CAD build for the part. Positions are in the model's coordinates, mm. A direction names the side the tool comes from. Round coordinates to 2 decimals unless told otherwise and drop trailing zeros. Write each loop counter-clockwise with the first axis right and the second up, starting at its lowest first coordinate (ties: lowest second). Pieces come first, ordered by that corner, then holes. Notation, with made-up numbers: (-16.5, 29.5) - (-3.5, 29.5) arc R5 cw to (-3.5, 37.5) - close; hole circle Ø10 at (11.5, -18). An arc over 180 degrees is marked (long way). Answer in a Markdown table with one row per item.
```python
from build123d import *

# Parameters (mm, degrees)
F0_W     = 58.42
F0_H     = 58.42
F1_DEPTH = 68.390979
F2_W     = 34.69379
F2_H     = 28.147937
F4_R     = 13.288258
F5_DEPTH = 140.97


with BuildPart() as f1:
    # F0 (on Top) → F1 (new body)
    with BuildSketch(Plane.XY):
        with Locations((-12.080159, 8.183077)):
            Rectangle(F0_W, F0_H)
    extrude(amount=F1_DEPTH)

    # F2 (on face) → F3 (revolve)
    with BuildSketch(Plane.XZ.offset(21.026923)):
        with Locations((-14.097282, 32.681106)):
            Rectangle(F2_W, F2_H)
    revolve(axis=Axis((17.129841, -21.026923, 34.195489), (0, 0, 1)))

    # F4 (on face) → F5 (cut)
    with BuildSketch(Plane.XY.offset(68.390979)):
        with Locations((-23.98462, 13.432804)):
            Circle(F4_R)
    extrude(amount=-F5_DEPTH, mode=Mode.SUBTRACT)


solid = f1.part
```
Q1. Flat gauge pins, fed straight in: pin 1 (22 mm diameter, centred on x = 17.13, y = -21.03, fed in from -Z); pin 2 (17.5 mm diameter, centred on y = -1.5, z = 45, fed in from +X); pin 3 (8 mm diameter, centred on y = -2, z = 23, fed in from +X); pin 4 (1.5 mm diameter, centred on x = 32.5, y = 7.5, fed in from +Z). Where does each tip first touch, or does it go through?
Computed:
| item | result |
|---|---|
| pin 1 | stops at z = 0 |
| pin 2 | stops at x = 64.49 |
| pin 3 | stops at x = 63.32 |
| pin 4 | stops at z = 46.76 |
Q2. Saw through at A-A on x = -29. List the corners of the cut face in (y, z).
Computed:
| item | result |
|---|---|
| outline | (-36.24, 18.61) - (-21.03, 18.61) - (-21.03, 0) - (1.13, 0) - (1.13, 68.39) - (-21.03, 68.39) - (-21.03, 46.76) - (-36.24, 46.76) - close; (25.74, 0) - (37.39, 0) - (37.39, 68.39) - (25.74, 68.39) - close |
Q3. Pull direction X, two halves, no side cores. Call faces 1 (the cylindrical face through (-34.53, 5.35, 34.67)), 2 (the cylindrical face through (50.325, -56.488, 32.878)), 3 (the flat face through (-41.29, 8, 34)): released by +X, released by -X, zero draft, split by the parting line, or undercut.
Computed:
| item | result |
|---|---|
| face 1 | undercut |
| face 2 | split by the parting line |
| face 3 | released by -X |
Q4. Saw through at D-D on z = 30.5. List the corners of the cut face in (x, y), then the cut area to 3 significant figures.
Computed:
| item | result |
|---|---|
| outline | (-41.29, -21.03) - (-31.44, -21.03) arc R48.57 ccw (long way) to (17.13, 27.55) - (17.13, 37.39) - (-41.29, 37.39) - close; hole circle Ø26.58 at (-23.98, 13.43); hole (3.25, -21.03) arc R13.88 ccw (long way) to (17.13, -7.15) - (17.13, -21.03) - close |
| area | 7,960 mm2 |
Q5. Drill centre lines: line 1 (Z direction, x = 57, y = -34); line 2 (Y direction, x = -12, z = 63.5); line 3 (X direction, y = -31, z = 45). Where is each one in solid material? Low to high.
Computed:
| item | result |
|---|---|
| line 1 | z = 18.61 to 46.76 |
| line 2 | y = -21.03 to 7.69, 19.17 to 37.39 |
| line 3 | x = -30.41 to 7.48, 26.78 to 64.67 |
Q6. 3-axis set-ups, long thin cutter, end or side, ignore diameter. For faces 4 (the flat face through (29, -33, 46.755)), 5 (the flat face through (-12, 37.393, 34)), 6 (the flat face through (29, -33, 18.607)): which of +Z, -Z, +X, -X, +Y, -Y reach the whole face in a straight line?
Computed:
| item | result |
|---|---|
| face 4 | +Z, +X, -Y |
| face 5 | +Z, -Z, +X, -X, +Y |
| face 6 | -Z, +X, -Y |
Q7. Saw through at C-C on z = 4. List the corners of the cut face in (x, y), then the cut area to 3 significant figures.
Computed:
| item | result |
|---|---|
| outline | (-41.29, -21.03) - (17.13, -21.03) - (17.13, 37.39) - (-41.29, 37.39) - close; hole circle Ø26.58 at (-23.98, 13.43) |
| area | 2,860 mm2 |
Q8. Saw through at B-B on y = 12. List the corners of the cut face in (x, z), then the cut area to 3 significant figures.
Computed:
| item | result |
|---|---|
| outline | (-41.29, 0) - (-37.2, 0) - (-37.2, 68.39) - (-41.29, 68.39) - close; (-10.77, 0) - (17.13, 0) - (17.13, 18.61) - (52.75, 18.61) - (52.75, 46.76) - (17.13, 46.76) - (17.13, 68.39) - (-10.77, 68.39) - close |
| area | 3,190 mm2 |
